Can you work these out from the model? Positions are in its coordinate system, mm. Face numbers are marked on the shaded views. A direction names the side the tool comes from. Give positions to 0.01 mm unless a question says otherwise; leave off trailing zeros. Order: outer loops, then holes, each group sorted by start corner. A loop starts at its lowest first (then second) coordinate and runs counter-clockwise, first axis right, second up. Notation, with made-up numbers: M 22,79 L 55,79 A13 cw 55,83 Z; hole C 50.5,-5 d9. An arc over 180 degrees is marked long. Use a Markdown table: item, result. Add a question column.
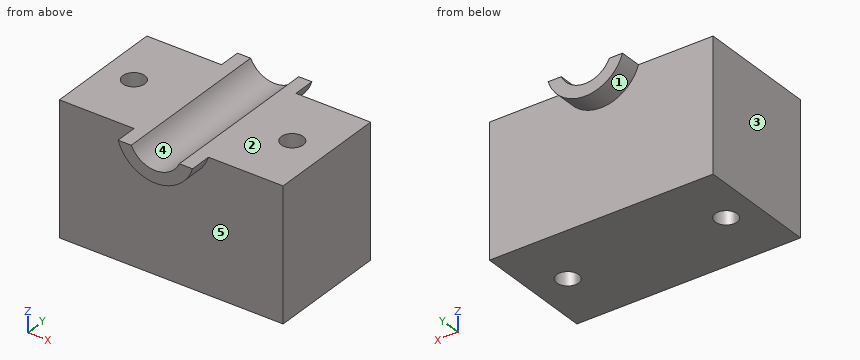
from build123d import *

# Parameters (mm, degrees)
F0_W     = 129.4137537479
F0_H     = 69.6472600102
F1_DEPTH = 76.2
F3_DEPTH = 12.7
F4_DEPTH = 127
F6_DEPTH = 12.7
F7_R     = 6.35
F8_DEPTH = 127


with BuildPart() as f1:
    # F0 (on Top) → F1 (new body)
    with BuildSketch(Plane.XY):
        Rectangle(F0_W, F0_H)
    extrude(amount=F1_DEPTH)

    # F2 (on face) → F3 (join)
    with BuildSketch(Plane(origin=(0, 34.8236300051, 0), x_dir=(-1, 0, 0), z_dir=(0, 1, 0))):
        with BuildLine():
            Line((-13.906876874, 76.2), (-21.526876874, 76.2))
            ThreePointArc((-21.526876874, 76.2), (0, 60.3776017268), (21.526876874, 76.2))
            Line((21.526876874, 76.2), (13.906876874, 76.2))
            ThreePointArc((13.906876874, 76.2), (0, 67.3132582233), (-13.906876874, 76.2))
        make_face()
    extrude(amount=F3_DEPTH)

    # F2 (on face) → F4 (cut)
    with BuildSketch(Plane(origin=(0, 34.8236300051, 0), x_dir=(-1, 0, 0), z_dir=(0, 1, 0))):
        with BuildLine():
            Line((13.906876874, 76.2), (-13.906876874, 76.2))
            ThreePointArc((-13.906876874, 76.2), (0, 67.3132582233), (13.906876874, 76.2))
        make_face()
    extrude(amount=-F4_DEPTH, mode=Mode.SUBTRACT)

    # F5 (on face) → F6 (join)
    with BuildSketch(Plane.XZ.offset(34.8236300051)):
        with BuildLine():
            Line((-13.906876874, 76.2), (-21.526876874, 76.2))
            ThreePointArc((-21.526876874, 76.2), (0, 60.3776017268), (21.526876874, 76.2))
            Line((21.526876874, 76.2), (13.906876874, 76.2))
            ThreePointArc((13.906876874, 76.2), (0, 67.3132582233), (-13.906876874, 76.2))
        make_face()
    extrude(amount=F6_DEPTH)

    # F7 (on face) → F8 (cut)
    with BuildSketch(Plane.XY.offset(76.2)):
        with Locations((-46.926876874, 0)):
            Circle(F7_R)
        with Locations((44.7043851018, 0)):
            Circle(F7_R)
    extrude(amount=-F8_DEPTH, mode=Mode.SUBTRACT)


solid = f1.part
1. If we section it at A-A, the plane y = 0: List the corners of the cut face in (x, z) for me, then the cut area to 3 significant figures.
2. Will these pins go through, and if not, where does the flat tip stop? pin 1 (3 mm diameter, centred on x = 23, z = 25.5, fed in from -Y); pin 2 (4 mm diameter, centred on x = -7.5, y = 18, fed in from +Z); pin 3 (8 mm diameter, centred on x = 4, y = -0.5, fed in from +Z).
3. On a 3-axis mill with a long thin cutter (end or side, diameter ignored), from which of +Z, -Z, +X, -X, +Y, -Y can I reach the whole of each face in a straight line? I mean the marked faces 1 and 2. Say none if no direction works.
4. We'd pull the mould along X, two halves only. Please class the marked faces 3, 4 and 5: +X half, -X half, draft (parallel to the pull), parting line (faces both ways), or undercut.
5. If we section it at C-C, the plane z = 24.5: List the corners of the cut face in (x, y) for me, then the cut area to 3 significant figures.
6. I need wall thicknesses on L1, parallel to Y at x = -34, z = 50; L2, parallel to X at y = -16.5, z = 73; L3, parallel to X at y = 5, z = 36. Which ranges of each line are inside material? Lowest first, please. Write a range as [from, to].
7. If we section it at D-D, the plane x = -48: List the corners of the cut face in (y, z) for me.
8. If we section it at B-B, the plane z = 70: List the corners of the cut face in (x, y) for me.
Geometry results:
| question | item | result |
|---|---|---|
| 1 | outline | M -64.71,0 L -53.28,0 L -53.28,76.2 L -64.71,76.2 Z; M -40.58,0 L 38.35,0 L 38.35,76.2 L 13.91,76.2 A15.32 cw -13.91,76.2 L -40.58,76.2 Z; M 51.05,0 L 64.71,0 L 64.71,76.2 L 51.05,76.2 Z |
| 1 | area | 7,750 mm^2 |
| 2 | pin 1 | stops at y = -34.82 |
| 2 | pin 2 | stops at z = 70.61 |
| 2 | pin 3 | stops at z = 69.57 |
| 3 | face 1 | -Z, +Y |
| 3 | face 2 | +Z, +X, -X, +Y, -Y |
| 4 | face 3 | -X half |
| 4 | face 4 | undercut |
| 4 | face 5 | draft |
| 5 | outline | M -64.71,-34.82 L 64.71,-34.82 L 64.71,34.82 L -64.71,34.82 Z; hole C -46.93,0 d12.7; hole C 44.7,0 d12.7 |
| 5 | area | 8,760 mm^2 |
| 6 | L1 | y = [-34.82, 34.82] |
| 6 | L2 | x = [-64.71, -11.91], [11.91, 64.71] |
| 6 | L3 | x = [-64.71, -50.84], [-43.01, 40.79], [48.62, 64.71] |
| 7 | outline | M -34.82,0 L -6.26,0 L -6.26,76.2 L -34.82,76.2 Z; M 6.26,0 L 34.82,0 L 34.82,76.2 L 6.26,76.2 Z |
| 8 | outline | M -64.71,-34.82 L -18.48,-34.82 L -18.48,-47.52 L -8.67,-47.52 L -8.67,47.52 L -18.48,47.52 L -18.48,34.82 L -64.71,34.82 Z; M 8.67,-47.52 L 18.48,-47.52 L 18.48,-34.82 L 64.71,-34.82 L 64.71,34.82 L 18.48,34.82 L 18.48,47.52 L 8.67,47.52 Z; hole C -46.93,0 d12.7; hole C 44.7,0 d12.7 |
